Verification items for the finished model (mm, model axes). A direction names the side the tool comes from. Round coordinates to 2 decimals unless told otherwise and drop trailing zeros. Write each loop counter-clockwise with the first axis right and the second up, starting at its lowest first coordinate (ties: lowest second). Pieces come first, ordered by that corner, then holes. Notation, with made-up numbers: M 72.25,-21 L 76.25,-21 A25 ccw 76.25,5 Z; hole C 89.5,57.25 d2. An arc over 180 degrees is marked long. One line per question, with ' | ' between items.
from build123d import *

# Parameters (mm, degrees)
BOX076_W               = 12
BOX076_H               = 3
BOX076_DEPTH           = 12
CYLINDER042_R          = 3.5
CYLINDER042_DEPTH      = 1
CYLINDER042_ROLL_ANGLE = 90


with BuildPart() as cube075:
    # Box076 → Box076 (new body)
    with BuildSketch(Plane(origin=(0, 71, 0), x_dir=(1, 0, 0), z_dir=(0, 0, 1))):
        with Locations((6, 1.5)):
            Rectangle(BOX076_W, BOX076_H)
    extrude(amount=BOX076_DEPTH)


with BuildPart() as obj1:
    # Cylinder042 → Cylinder042 (new body)
    with BuildSketch(Plane.XY):
        Circle(CYLINDER042_R)
    extrude(amount=CYLINDER042_DEPTH)


with BuildPart() as obj1_1:
    # Cylinder042 roll: moved
    add(obj1.part.rotate(Axis((0, 0, 0), (1, 0, 0)), CYLINDER042_ROLL_ANGLE))


with BuildPart() as obj1_2:
    # Cylinder042 placement: moved
    add(obj1_1.part.moved(Location((6, 75, 6))))

    # Fusion024: union Cube075
    add(cube075.part)


with BuildPart() as obj1_3:
    # Fusion024 placement: moved
    add(obj1_2.part.moved(Location((44, -12.5, 47))))


solid = obj1_3.part
1. Section check B-B, the plane z = 53. Record the cut outline in (x, y), then the cut area to 3 significant figures.
Results:
outline: M 44,58.5 L 56,58.5 L 56,61.5 L 53.5,61.5 L 53.5,62.5 L 46.5,62.5 L 46.5,61.5 L 44,61.5 Z | area: 43.0 mm2
2. Thickness scan on line 1 (Y direction, x = 50, z = 49.25); line 2 (X direction, y = 62.3, z = 53.5); line 3 (X direction, y = 62.2, z = 52.25). Record the ranges inside material, lowest first.
Results:
line 1: y = 58.5 to 61.5 | line 2: x = 46.54 to 53.46 | line 3: x = 46.58 to 53.42
3. Section check D-D, the plane x = 46. Record the cut outline in (y, z), then the cut area to 3 significant figures.
Results:
outline: M 58.5,47 L 61.5,47 L 61.5,59 L 58.5,59 Z | area: 36.0 mm2
4. Go/stop test with a flat-tipped pin: P1, Ø6, axis at x = 53, z = 49.5, coming from the +Y side. Record where the tip stops, or that it passes through.
Results:
P1: stops at y = 62.5
5. Tool access check on faces 1 (the face through (50, 60, 47)), 2 (the face through (53, 61.5, 56)). Record the directions out of +Z, -Z, +X, -X, +Y, -Y that give a thin tool (end or side, any length) a straight path to the whole face; none if there is none.
Results:
face 1: -Z, +X, -X, +Y, -Y | face 2: +Y
6. Section check C-C, the plane z = 49.25. Record the cut outline in (x, y), then the cut area to 3 significant figures.
Results:
outline: M 44,58.5 L 56,58.5 L 56,61.5 L 44,61.5 Z | area: 36.0 mm2
7. Section check A-A, the plane x = 50. Record the cut outline in (y, z), then the cut area to 3 significant figures.
Results:
outline: M 58.5,47 L 61.5,47 L 61.5,49.5 L 62.5,49.5 L 62.5,56.5 L 61.5,56.5 L 61.5,59 L 58.5,59 Z | area: 43.0 mm2
